from build123d import *

# Parameters (mm, degrees)
F1_DEPTH = 6.35
F3_D     = 38.1
F3_DEPTH = 6.35
F3_TIP   = 11.4463947925
F4_D     = 8.4328


with BuildPart() as f1:
    # F0 (on Right) → F1 (new body)
    with BuildSketch(Plane.YZ):
        with BuildLine():
            Line((63.5, 15.875), (0, 31.75))
            ThreePointArc((0, 31.75), (-31.75, 0), (0, -31.75))
            Line((0, -31.75), (63.5, -15.875))
            ThreePointArc((63.5, -15.875), (79.375, 0), (63.5, 15.875))
        make_face()
    extrude(amount=F1_DEPTH)

    # F3
    with Locations(Plane.YZ.offset(6.35)):
        with Locations((0, 0)):
            Hole(F3_D / 2, depth=F3_DEPTH)
            with Locations((0, 0, -(F3_DEPTH + F3_TIP / 2))):  # 118° drill point
                Cone(0, F3_D / 2, F3_TIP, mode=Mode.SUBTRACT)

    # F4 (through all)
    with Locations(Plane.YZ.offset(6.35)):
        with Locations((63.5, 0)):
            Hole(F4_D / 2)


solid = f1.part
Design review of the part built by this model. Coordinates are the model's own, in mm. Coordinates: 2 decimals unless noted, no trailing zeros. Write each loop counter-clockwise with the first axis right and the second up, starting at its lowest first coordinate (ties: lowest second). Pieces come first, ordered by that corner, then holes. Notation, with made-up numbers: (-6.5, -31.75) - (13.5, -31.75) arc R19 cw to (13.5, -23.75) - close; hole circle Ø10 at (29.25, 65). An arc over 180 degrees is marked (long way). One line per item, written item: value.
1) Add section D-D (z = -22). State the section outline as (x, y) points, plus the area to 3 significant figures.
Answer sheet:
outline: (0, -22.89) - (6.35, -22.89) - (6.35, 39) - (0, 39) - close
area: 393 mm2
2) Insertion check: pin 1 (2 mm diameter, centred on x = 3, y = 34.5, fed in from +Z) (3 decimals); pin 2 (7.5 mm diameter, centred on y = 63.5, z = 0, fed in from -X); pin 3 (1 mm diameter, centred on x = 4.5, z = 20, fed in from -Y). Each pin has a flat end and moves straight along its axis. Give the tip position at first contact, or say it passes through.
Answer sheet:
pin 1: stops at z = 23.375
pin 2: passes through
pin 3: stops at y = -25.06
3) Mouldability with a two-part tool opening along Y and no side actions: class faces 1 (the face through (3.13, 79.37, -0.35)), 2 (the face through (3.131, -31.742, 0.698)), 3 (the face through (6.35, 23, 0)), 4 (the face through (3.131, 67.712, 0.185)) as +Y half, -Y half, draft (parallel to the pull), parting line (faces both ways), or undercut.
Answer sheet:
face 1: +Y half
face 2: -Y half
face 3: draft
face 4: undercut
4) Add section C-C (x = 5). State the section outline as (y, z) points (3 decimals).
Answer sheet:
outline: (0, -31.75) - (63.5, -15.875) arc R15.875 ccw to (63.5, 15.875) - (0, 31.75) arc R31.75 ccw to start; hole circle Ø38.1 at (0, 0); hole circle Ø8.433 at (63.5, 0)
5) Add section B-B (y = 7). State the section outline as (x, z) points, plus the area to 3 significant figures.
Answer sheet:
outline: (0, -30) - (6.35, -30) - (6.35, -17.72) - (0, -17.72) - close; (0, 17.72) - (6.35, 17.72) - (6.35, 30) - (0, 30) - close
area: 156 mm2
6) Add section A-A (z = 0). State the section outline as (x, y) points (3 decimals).
Answer sheet:
outline: (0, -31.75) - (6.35, -31.75) - (6.35, -19.05) - (0, -19.05) - close; (0, 19.05) - (6.35, 19.05) - (6.35, 59.284) - (0, 59.284) - close; (0, 67.716) - (6.35, 67.716) - (6.35, 79.375) - (0, 79.375) - close
7) To check wall thickness, follow probe 1 along Z at (x, y) = (1.75, 0); probe 2 along Z at (x, y) = (2, 63.5) (3 decimals); probe 3 along Y at (x, z) = (5.75, 2.5). State the ranges of each line that lie inside material, in increasing order.
Answer sheet:
probe 1: z = -31.75 to -19.05, 19.05 to 31.75
probe 2: z = -15.875 to -4.216, 4.216 to 15.875
probe 3: y = -31.65 to -18.89, 18.89 to 60.1, 66.9 to 79.18
